Can you work these out from the model? Positions are in its coordinate system, mm. A direction names the side the tool comes from. Give positions to 0.01 mm unless a question says otherwise; leave off trailing zeros. Loops run counter-clockwise (first coordinate to the right, second up) from the corner with the lowest first, then second, coordinate; pieces in that order, holes last. Notation, with made-up numbers: M 85.5,22 L 129.5,22 A9 ccw 129.5,28 Z; hole C 17.5,44.5 d7. An arc over 180 degrees is marked long. Use CSV: the item, a comma, the result in double quotes.
from build123d import *

# Parameters (mm, degrees)
F0_R     = 20
F1_DEPTH = 50
F2_R     = 27.5
F2_R_2   = 20
F3_DEPTH = 35
F4_R     = 29.753541
F4_R_2   = 22.5
F5_DEPTH = 15


with BuildPart() as f1:
    # F0 (on Front) → F1 (new body)
    with BuildSketch(Plane.XZ):
        Circle(F0_R)
        with BuildLine():
            ThreePointArc((3.875362, 14.490741), (11.898118, 9.134264), (15, 0))
            ThreePointArc((15, 0), (11.898118, -9.134264), (3.875362, -14.490741))
            ThreePointArc((3.875362, -14.490741), (0, -17.5), (-3.875362, -14.490741))
            ThreePointArc((-3.875362, -14.490741), (-15, 0), (-3.875362, 14.490741))
            ThreePointArc((-3.875362, 14.490741), (0, 17.5), (3.875362, 14.490741))
        make_face(mode=Mode.SUBTRACT)
    extrude(amount=F1_DEPTH)

    # F2 (on face) → F3 (join)
    with BuildSketch(Plane.XZ.offset(50)):
        Circle(F2_R)
        Circle(F2_R_2, mode=Mode.SUBTRACT)
    extrude(amount=-F3_DEPTH)

    # F4 (on face) → F5 (cut)
    with BuildSketch(Plane.XZ.offset(50)):
        Circle(F4_R)
        Circle(F4_R_2, mode=Mode.SUBTRACT)
    extrude(amount=-F5_DEPTH, mode=Mode.SUBTRACT)


solid = f1.part
Q1. I want a section at B-B, the plane y = -14. Please give me the cut outline in (x, z).
Model answer:
outline,"C 0,0 d40; hole M -3.88,-14.49 A4 ccw 3.88,-14.49 A15 ccw 15,0 A15 ccw 3.88,14.49 A4 ccw -3.88,14.49 A15 ccw Z"
Q2. I want a section at A-A, the plane x = 0. Please give me the cut outline in (y, z), then the cut area to 3 significant figures.
Model answer:
outline,"M -50,-22.5 L -35,-22.5 L -35,-27.5 L -15,-27.5 L -15,-20 L 0,-20 L 0,-17.5 L -50,-17.5 Z; M -50,17.5 L 0,17.5 L 0,20 L -15,20 L -15,27.5 L -35,27.5 L -35,22.5 L -50,22.5 Z"
area,"625 mm2"
Q3. I want a section at C-C, the plane z = 1.5. Please give me the cut outline in (x, y).
Model answer:
outline,"M -27.46,-35 L -22.45,-35 L -22.45,-50 L -14.92,-50 L -14.92,0 L -19.94,0 L -19.94,-15 L -27.46,-15 Z; M 14.92,-50 L 22.45,-50 L 22.45,-35 L 27.46,-35 L 27.46,-15 L 19.94,-15 L 19.94,0 L 14.92,0 Z"
Q4. I'm going to push flat-ended pins straight in: P1, Ø1.5, axis at y = -8.5, z = -8, coming from the -X side; P2, Ø2, axis at x = 19, z = -21, coming from the +Y side; P3, Ø5, axis at x = -18.5, y = -21, coming from the +Z side; P4, Ø8, axis at x = -1, z = -9, coming from the -Y side. Where does each tip first touch, or does it pass through?
Model answer:
P1,"x = -18.64"
P2,"y = -15"
P3,"z = 22.37"
P4,"through"
Q5. I want a section at D-D, the plane z = -18.5. Please give me the cut outline in (x, y).
Model answer:
outline,"M -20.35,-35 L -12.81,-35 L -12.81,-50 L 12.81,-50 L 12.81,-35 L 20.35,-35 L 20.35,-15 L 7.6,-15 L 7.6,0 L -7.6,0 L -7.6,-15 L -20.35,-15 Z"
Q6. If we mould it in two halves opening along Z, with no side actions, what happens to faces 1 (the cylindrical face through (10.382, -42.605, -19.961)), 2 (the cylindrical face through (-15, -25, 0)), 3 (the cylindrical face through (0.1, -24.6, -17.5)), 4 (the flat face through (5, -50, -15))? For each: released by +Z, released by -Z, zero draft, split by the parting line, or undercut.
Model answer:
face 1,"split by the parting line"
face 2,"undercut"
face 3,"undercut"
face 4,"zero draft"
Q7. For faces 5 (the flat face through (1.9, -15, -20.2)), 6 (the flat face through (-23, -35, 0)), 7 (the flat face through (-5, 0, -15)), 8 (the cylindrical face through (-0.1, -24.6, 17.5)), which set-ups out of +Z, -Z, +X, -X, +Y, -Y let a thin tool reach every point of the face, with its end or its side?
Model answer:
face 5,"+Y"
face 6,"-Y"
face 7,"+Z, -Z, +X, -X, +Y"
face 8,"+Y, -Y"
Q8. Please list where these lines run through material, in increasing order: L1, parallel to Y at x = 24, z = 13; L2, parallel to X at y = -37.5, z = -0.5; L3, parallel to Z at x = 0, y = -23. Write a range as from..to.
Model answer:
L1,"-35..-15"
L2,"-22.49..-14.99, 14.99..22.49"
L3,"-27.5..-17.5, 17.5..27.5"
